Study the drawing (mm; zero at the part's minimum x, y, z) and answer. Coordinates: 2 decimals unless noted, no trailing zeros. Write each loop counter-clockwise with the first axis right and the second up, starting at its lowest first coordinate (ties: lowest second). Pieces come first, ordered by that corner, then holes. Notation, with made-up numbers: M 11.5,89.25 L 37.5,89.25 A24 ccw 37.5,114.25 Z; hole C -4.75,50 d11. An arc over 180 degrees is marked long. Answer as a JSON object with one key per item and string values. Group by question number.
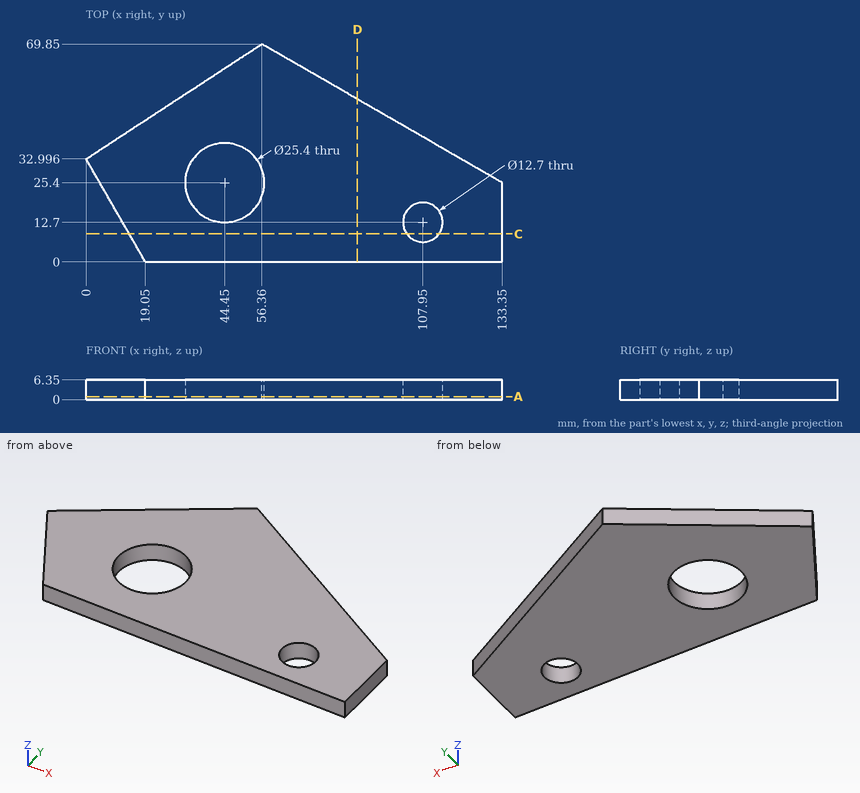
Item 1: A cutting plane is placed at C-C, the plane y = 9. Write down the section's boundary in (x, z).
Item 2: A cutting plane is placed at D-D, the plane x = 87. Write down the section's boundary in (y, z), and give its area (3 significant figures).
Item 3: Consider L1, parallel to X at y = 15, z = 0.75; L2, parallel to Y at x = 44.45, z = 4.5; L3, parallel to Y at x = 110.5, z = 5.5 (1 decimal). Determine where each line is inside the solid, lowest interval first. Write a range as from..to.
Item 4: A cutting plane is placed at A-A, the plane z = 1. State how many separate pieces and enclosed holes the cut face has, and give its area (3 significant figures).
Item 5: Flat-ended cylindrical pins translate along their axes: pin 1 Ø1.5 at (y, z) = (14.5, 5.5) entering from -X (1 decimal); pin 2 Ø7.5 at (x, y) = (107.95, 12.7) entering from -Z. Find the tip coordinate at first contact, or state that the pin passes through.
Answer:
{
 "1": {"outline": "M 13.85,0 L 102.79,0 L 102.79,6.35 L 13.85,6.35 Z; M 113.11,0 L 133.35,0 L 133.35,6.35 L 113.11,6.35 Z"},
 "2": {"outline": "M 0,0 L 52.16,0 L 52.16,6.35 L 0,6.35 Z", "area": "331 mm2"},
 "3": {"L1": "10.39..37.16, 51.74..102.03, 113.87..133.35", "L2": "0..12.7, 38.1..62.06", "L3": "0..6.9, 18.5..38.6"},
 "4": {"separate pieces": "1", "enclosed holes": "2", "area": "5,620 mm2"},
 "5": {"pin 1": "x = 10.2", "pin 2": "through"}
}
